from build123d import *

# Parameters (mm, degrees)
F0_W     = 190.5
F0_H     = 19.05
F1_DEPTH = 6.35
F3_D     = 8.4328
F5_DEPTH = 190.501


with BuildPart() as f1:
    # F0 (on Front) → F1 (new body)
    with BuildSketch(Plane.XZ):
        with Locations((95.25, 9.525)):
            Rectangle(F0_W, F0_H)
    extrude(amount=F1_DEPTH)

    # F3 (through all)
    with Locations(Plane.XZ.offset(6.35)):
        with Locations((11.74115, 6.92785), (67.72275, 6.92785), (123.70435, 6.92785), (179.80025, 6.92785)):
            Hole(F3_D / 2)

    # F4 (on face) → F5 (cut, through all)
    with BuildSketch(Plane.YZ.offset(190.5)):
        Polygon((-6.35, 19.05), (-6.35, 12.0396), (-3.4036, 12.0396), (-3.8862, 19.05), align=None)
    extrude(amount=-F5_DEPTH, mode=Mode.SUBTRACT)


solid = f1.part
Check sheet for the modelled part. Datum: model origin and axes. Units: mm. A direction names the side the tool comes from. Coordinates: 2 decimals unless noted, no trailing zeros. Loops run counter-clockwise (first coordinate to the right, second up) from the corner with the lowest first, then second, coordinate; pieces in that order, holes last. Notation, with made-up numbers: (-2, -28.75) -> (31, -28.75) arc R23 ccw to (31, -11.75) -> close; hole circle Ø1 at (59.5, 52.25). An arc over 180 degrees is marked (long way). Answer in a Markdown table with one row per item.
1. Sectioned sample at A-A, the plane y = -5. Record the boundary of the cut face in (x, z), then the cut area to 3 significant figures.
Check values:
| item | result |
|---|---|
| outline | (0, 0) -> (190.5, 0) -> (190.5, 12.04) -> (0, 12.04) -> close; hole circle Ø8.43 at (11.74, 6.93); hole circle Ø8.43 at (67.72, 6.93); hole circle Ø8.43 at (123.7, 6.93); hole circle Ø8.43 at (179.8, 6.93) |
| area | 2,070 mm2 |
2. Sectioned sample at B-B, the plane x = 123.5. Record the boundary of the cut face in (y, z).
Check values:
| item | result |
|---|---|
| outline | (-6.35, 0) -> (0, 0) -> (0, 2.72) -> (-6.35, 2.72) -> close; (-6.35, 11.14) -> (0, 11.14) -> (0, 19.05) -> (-3.89, 19.05) -> (-3.4, 12.04) -> (-6.35, 12.04) -> close |
3. Sectioned sample at C-C, the plane z = 15.75. Record the boundary of the cut face in (x, y), then the cut area to 3 significant figures.
Check values:
| item | result |
|---|---|
| outline | (0, -3.66) -> (190.5, -3.66) -> (190.5, 0) -> (0, 0) -> close |
| area | 697 mm2 |
4. Material ranges on line 1 along X through (y, z) = (-1.5, 6.5); line 2 along X through (y, z) = (-5.25, 3.5); line 3 along Z through (x, y) = (173.5, -5.5), recorded low to high. Write a range as [from, to].
Check values:
| item | result |
|---|---|
| line 1 | x = [0, 7.55], [15.94, 63.53], [71.92, 119.51], [127.9, 175.61], [183.99, 190.5] |
| line 2 | x = [0, 9.29], [14.2, 65.27], [70.18, 121.25], [126.16, 177.35], [182.26, 190.5] |
| line 3 | z = [0, 12.04] |
5. Release check for a two-part mould opening along X. For faces 3 (the face through (71.935, -3.131, 7.113)), 4 (the face through (119.68, -3.13, 8.19)), 5 (the face through (190.5, -3, 7)), 6 (the face through (97, -5, 12.04)) record: released by +X, released by -X, zero draft, split by the parting line, or undercut.
Check values:
| item | result |
|---|---|
| face 3 | undercut |
| face 4 | undercut |
| face 5 | released by +X |
| face 6 | zero draft |
6. Go/stop test with flat-tipped pins: pin 1 (9.5 mm diameter, centred on x = 67.72, z = 6.93, fed in from +Y); pin 2 (5 mm diameter, centred on x = 123.7, z = 6.93, fed in from +Y); pin 3 (3 mm diameter, centred on x = 144.5, z = 16.5, fed in from -Y). Record where each tip stops, or that it passes through.
Check values:
| item | result |
|---|---|
| pin 1 | stops at y = 0 |
| pin 2 | passes through |
| pin 3 | stops at y = -3.81 |
7. Access from +Z, -Z, +X, -X, +Y, -Y to the whole of each face (thin tool, end or side, straight path). Record for faces 1 (the face through (96.58, -3.64, 15.5)), 2 (the face through (0, -3, 7)).
Check values:
| item | result |
|---|---|
| face 1 | +X, -X, -Y |
| face 2 | +Z, -Z, -X, +Y, -Y |
